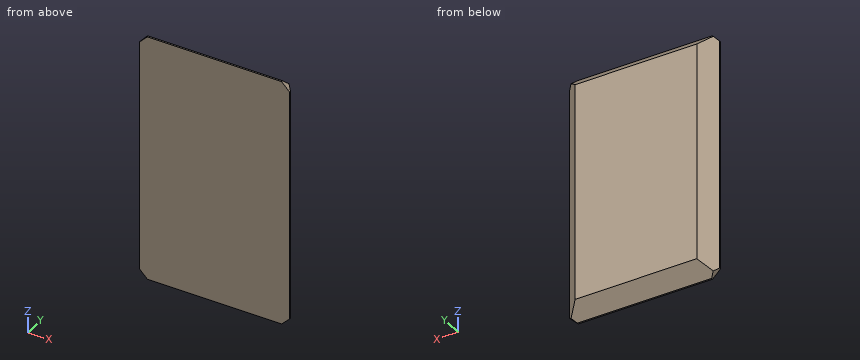
Autodesk Inventor part; units mm, degrees
ref_plane "YZ Plane" through (0, 0, 0) normal (1, 0, 0) x (0, 1, 0)
ref_plane "XZ Plane" through (0, 0, 0) normal (0, 1, 0) x (-1, 0, 0)
ref_plane "XY Plane" through (0, 0, 0) normal (0, 0, 1) x (1, 0, 0)
sketch "Эскиз1" plane through (0, 0, 0) normal (0, 1, 0) x (-1, 0, 0)
  line L0 (-47.5, 79) -> (47.5, 79)
  line L1 (47.5, 79) -> (47.5, -79)
  line L2 (47.5, -79) -> (-47.5, -79)
  line L3 (-47.5, -79) -> (-47.5, 79)
  line L4 (-47.5, 79) -> (47.5, -79) construction
  line L5 (47.5, 79) -> (-47.5, -79) construction
  point P0 (0, 0)
  dimension "d0" = 95
  dimension "d1" = 158
extrude "Выдавливание1" add sketch "Эскиз1" along normal blind 10
chamfer "Фаска1" distance 5 angle 45 1 edges at (47.5, 5, 79) measured on face at (47.5, 6.6667, 26.3333)
chamfer "Фаска2" distance 5 angle 45 1 edges at (47.5, 5, -79) measured on face at (15.8333, 3.3333, -79)
chamfer "Фаска3" distance 5 angle 45 1 edges at (-47.5, 5, -79) measured on face at (12.5, 3.3333, -79)
chamfer "Фаска4" distance 5 angle 45 1 edges at (-47.5, 5, 79) measured on face at (-17.5, 3.3333, 79)
chamfer "Фаска5" distance 9 angle 45 1 edges at (-47.5, 10, 0) measured on face at (15.8333, 10, 24.6667)
chamfer "Фаска6" distance 9 angle 45 1 edges at (2, 10, -79) measured on face at (-9.8333, 10, -24.6667)
chamfer "Фаска7" distance 9 angle 45 1 edges at (47.5, 10, 2) measured on face at (-9.8333, 10, 27.6667)
chamfer "Фаска8" distance 9 angle 45 1 edges at (0, 10, 79) measured on face at (12.8333, 10, -20.3333)
Could you check a few things on this model? Use its own coordinates, in mm. Round coordinates to 2 decimals unless told otherwise and drop trailing zeros. Loops run counter-clockwise (first coordinate to the right, second up) from the corner with the lowest first, then second, coordinate; pieces in that order, holes last. Notation, with made-up numbers: (50.5, 1.25) -> (93.5, 1.25) arc R33 ccw to (93.5, 31.25) -> close; hole circle Ø9 at (24, 15.25). An arc over 180 degrees is marked (long way). Put each result on its own line as item: value.
Q1. I want a section at B-B on y = 7.5. Write out the boundary of the cut face in (x, z).
Checks:
outline: (-41, -72.5) -> (41, -72.5) -> (41, 72.5) -> (-41, 72.5) -> close
Q2. I want a section at A-A on z = -33.5. Write out the boundary of the cut face in (x, y), and give its area (3 significant figures).
Checks:
outline: (-47.5, 0) -> (47.5, 0) -> (47.5, 1) -> (38.5, 10) -> (-38.5, 10) -> (-47.5, 1) -> close
area: 869 mm2
Q3. I want a section at C-C on x = -37. Write out the boundary of the cut face in (y, z).
Checks:
outline: (0, -79) -> (1, -79) -> (10, -70) -> (10, 70) -> (1, 79) -> (0, 79) -> close
Q4. Please list where these lines run through material, in increasing order: line 1 (Z direction, x = -39.5, y = 3.5); line 2 (Z direction, x = -9.5, y = 5.25); line 3 (X direction, y = 6.5, z = -12). Write a range as from..to.
Checks:
line 1: -76.5..76.5
line 2: -74.75..74.75
line 3: -42..42
Q5. For pin 1 Ø5 at (y, z) = (7, 54) entering from +X; pin 2 Ø2 at (x, y) = (14.5, 5) entering from +Z; pin 3 Ø6 at (y, z) = (2.5, 24) entering from -X; pin 4 Ø2 at (y, z) = (3.5, -53) entering from -X, each with a flat end and sliding along its axis, tell me the tip position at first contact or that it passes through.
Checks:
pin 1: x = 44
pin 2: z = 76
pin 3: x = -47.5
pin 4: x = -46
